Design review of the part built by this model. Coordinates are the model's own, in mm. Face numbers are marked on the shaded views. Give positions to 0.01 mm unless a question says otherwise; leave off trailing zeros. Order: outer loops, then holes, each group sorted by start corner. A loop starts at its lowest first (then second) coordinate and runs counter-clockwise, first axis right, second up. Notation, with made-up numbers: (-6.75, 74.25) -> (26.25, 74.25) arc R11 ccw to (26.25, 78.25) -> close; hole circle Ø9 at (-10.75, -28.75). An arc over 180 degrees is marked (long way). Return JSON: item names as keys, results as strings.
```python
from build123d import *

# Parameters (mm, degrees)
SKETCH1_R           = 2.38125
BOSS_EXTRUDE1_DEPTH = 7.62
SKETCH2_R           = 4.7625
BOSS_EXTRUDE2_DEPTH = 1.524
FILLET1_R           = 0.254
FILLET2_R           = 0.381
FILLET3_R           = 0.127
FILLET4_R           = 3.81
SKETCH4_R           = 1.27
CUT_EXTRUDE1_DEPTH  = 2.54
FILLET5_R           = 0.635


with BuildPart() as part:
    # Sketch1 → Boss-Extrude1 (new body)
    with BuildSketch(Plane(origin=(0, 0, 0), x_dir=(1, 0, 0), z_dir=(0, 1, 0))):
        Circle(SKETCH1_R)
    extrude(amount=BOSS_EXTRUDE1_DEPTH)

    # Sketch2 → Boss-Extrude2 (add)
    with BuildSketch(Plane(origin=(0, 7.62, 0), x_dir=(1, 0, 0), z_dir=(0, 1, 0))):
        Circle(SKETCH2_R)
    extrude(amount=BOSS_EXTRUDE2_DEPTH)

    # Fillet1
    fillet1_edges = [part.edges().sort_by_distance(p)[0] for p in [
        (-2.38125, 0, 0),
    ]]
    fillet(fillet1_edges, radius=FILLET1_R)

    # Sketch3 → Cut-Revolve1 (revolve, cut)
    with BuildSketch(Plane(origin=(0, 0, 0), x_dir=(0, 0, -1), z_dir=(1, 0, 0))):
        Polygon((-2.38125, 9.144), (-4.7625, 8.382), (-4.7625, 9.144), align=None)
    revolve(axis=Axis((0, 9.144, 0), (0, -1, 0)), mode=Mode.SUBTRACT)

    # Fillet2
    fillet2_edges = [part.edges().sort_by_distance(p)[0] for p in [
        (3.367596045, 8.382, 3.367596045),
    ]]
    fillet(fillet2_edges, radius=FILLET2_R)

    # Fillet3
    fillet3_edges = [part.edges().sort_by_distance(p)[0] for p in [
        (-4.7625, 7.62, 0),
    ]]
    fillet(fillet3_edges, radius=FILLET3_R)

    # Fillet4
    fillet4_edges = [part.edges().sort_by_distance(p)[0] for p in [
        (0, 9.144, -2.38125),
    ]]
    fillet(fillet4_edges, radius=FILLET4_R)

    # Sketch4 → Cut-Extrude1 (cut)
    with BuildSketch(Plane(origin=(0, 9.144, 0), x_dir=(1, 0, 0), z_dir=(0, 1, 0))):
        Circle(SKETCH4_R)
    extrude(amount=-CUT_EXTRUDE1_DEPTH, mode=Mode.SUBTRACT)

    # Fillet5
    fillet5_edges = [part.edges().sort_by_distance(p)[0] for p in [
        (-1.27, 6.604, 0),
    ]]
    fillet(fillet5_edges, radius=FILLET5_R)


solid = part.part
```
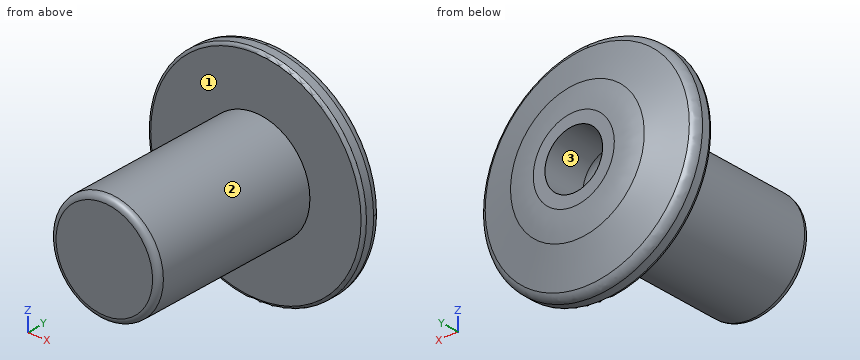
Item 1: Wall thickness on L1, parallel to Z at x = 0, y = 8; L2, parallel to Z at x = 0, y = 4.25: over which ranges is each line inside the solid? List them lowest first. Write a range as [from, to].
Result set:
{"L1": "z = [-4.76, -1.27], [1.27, 4.76]", "L2": "z = [-2.38, 2.38]"}
Item 2: Mouldability with a two-part tool opening along X and no side actions: class the marked faces 1, 2 and 3 as released by +X, released by -X, zero draft, split by the parting line, or undercut.
Result set:
{"face 1": "zero draft", "face 2": "split by the parting line", "face 3": "undercut"}
Item 3: Add section A-A (y = 3.5). Give the boundary of the cut face in (x, z), plus the area to 3 significant figures.
Result set:
{"outline": "circle Ø4.76 at (0, 0)", "area": "17.8 mm^2"}
Item 4: For pin 1 (1.5 mm diameter, centred on x = 2.5, z = -1.5, fed in from -Y); pin 2 (0.6 mm diameter, centred on x = -0.5, z = 0, fed in from +Y); pin 3 (1 mm diameter, centred on x = -1, y = 1, fed in from -Z), all flat-tipped, find the tip position at first contact; note any pin that passes through.
Result set:
{"pin 1": "stops at y = 0", "pin 2": "stops at y = 6.63", "pin 3": "stops at z = -2.33"}
